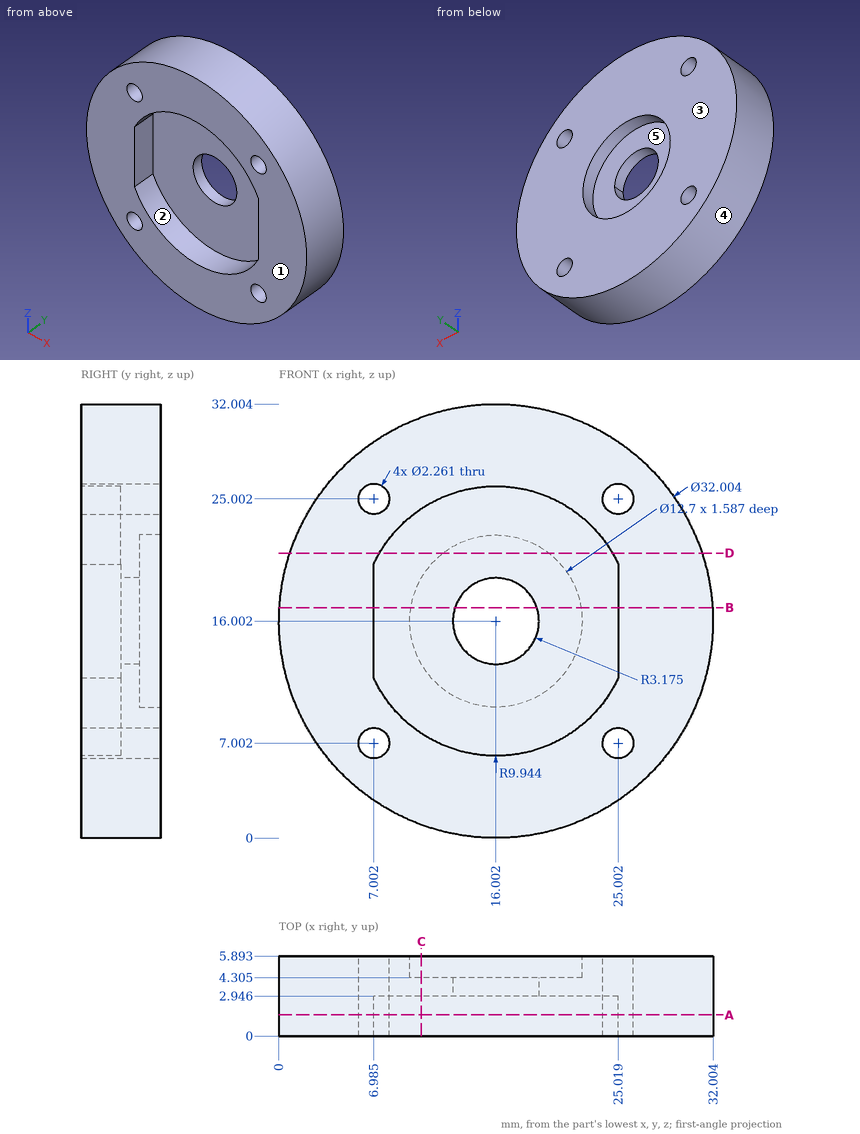
Design review of the part shown in the three views and the two pictorial views. Dimensions are in mm from the part's minimum x, y and z. A direction names the side the tool comes from. Coordinates: 2 decimals unless noted, no trailing zeros. Order: outer loops, then holes, each group sorted by start corner. A loop starts at its lowest first (then second) coordinate and runs counter-clockwise, first axis right, second up. Notation, with made-up numbers: (17, 14.5) -> (73, 14.5) arc R20 cw to (73, 24.5) -> close; hole circle Ø7 at (78, 74.5). An arc over 180 degrees is marked (long way). Use one line per item in the form item = value. Start each with the question number.
(1) Add section A-A on y = 1.55. State the section outline as (x, z) points (1 decimal), plus the area to 3 significant figures.
(2) Insertion check: pin 1 (1.5 mm diameter, centred on y = 2, z = 14, fed in from +X) (1 decimal); pin 2 (2 mm diameter, centred on x = 25, z = 25, fed in from +Y); pin 3 (2 mm diameter, centred on x = 14.5, y = 3, fed in from +Z); pin 4 (6.5 mm diameter, centred on x = 16, z = 14.5, fed in from +Y) (1 decimal). Each pin has a flat end and moves straight along its axis. Give the tip position at first contact, or say it passes through.
(3) Add section B-B on z = 17. State the section outline as (x, y) points (1 decimal).
(4) For the marked faces 1 and 2, list the 3-axis set-ups (+Z, -Z, +X, -X, +Y, -Y) from which the entire face can be reached by the end or side of a thin tool; tool diameter is ignored.
(5) Add section C-C on x = 10.5. State the section outline as (y, z) points (1 decimal), plus the area to 3 significant figures.
(6) The part is to be moulded in two halves that separate along X. For the marked faces 3, 4 and 5, say which applies: +X half, -X half, draft (parallel to the pull), parting line (faces both ways), or undercut.
(7) For probe 1 along X at (y, z) = (1.4, 15.5) (1 decimal); probe 2 along X at (y, z) = (0.95, 22) (1 decimal); probe 3 along Z at (x, y) = (6.5, 3.35) (1 decimal), list the stretches that pass through material, from the lowest coordinate up.
(8) Add section D-D on z = 21. State the section outline as (x, y) points (1 decimal).
Answer block:
q1.outline = circle Ø32 at (16, 16); hole circle Ø2.3 at (7, 7); hole circle Ø2.3 at (7, 25); hole (7, 11.8) arc R9.9 ccw to (25, 11.8) -> (25, 20.2) arc R9.9 ccw to (7, 20.2) -> close; hole circle Ø2.3 at (25, 7); hole circle Ø2.3 at (25, 25)
q1.area = 488 mm²
q2.pin_1 = 32
q2.pin_2 = through
q2.pin_3 = 32
q2.pin_4 = 4.3
q3.outline = (0, 0) -> (7, 0) -> (7, 2.9) -> (13, 2.9) -> (13, 4.3) -> (9.7, 4.3) -> (9.7, 5.9) -> (0, 5.9) -> close; (19, 2.9) -> (25, 2.9) -> (25, 0) -> (32, 0) -> (32, 5.9) -> (22.3, 5.9) -> (22.3, 4.3) -> (19, 4.3) -> close
q4.face_1 = +Z, -Z, +X, -X, -Y
q4.face_2 = -Y
q5.outline = (0, 1) -> (5.9, 1) -> (5.9, 12.8) -> (4.3, 12.8) -> (4.3, 19.2) -> (5.9, 19.2) -> (5.9, 31) -> (0, 31) -> (0, 24.3) -> (2.9, 24.3) -> (2.9, 7.7) -> (0, 7.7) -> close
q5.area = 118 mm²
q6.face_3 = draft
q6.face_4 = parting line
q6.face_5 = undercut
q7.probe_1 = 0 to 7, 25 to 32
q7.probe_2 = 1.2 to 8.1, 23.9 to 30.8
q7.probe_3 = 3.1 to 6, 8 to 24, 26 to 28.9
q8.outline = (0.8, 0) -> (7.4, 0) -> (7.4, 2.9) -> (24.6, 2.9) -> (24.6, 0) -> (31.2, 0) -> (31.2, 5.9) -> (19.9, 5.9) -> (19.9, 4.3) -> (12.1, 4.3) -> (12.1, 5.9) -> (0.8, 5.9) -> close
